Could you check a few things on this model? Use its own coordinates, in mm. A direction names the side the tool comes from. Round coordinates to 2 decimals unless told otherwise and drop trailing zeros. One line per question, with ' | ' between items. Start each with the question number.
1. If I drill on line 1 along Y through (x, z) = (80, 16); line 2 along Y through (x, z) = (-80, 14); line 3 along Z through (x, y) = (34, -32), over which ranges is the centre line in solid material (lowest first)? Write a range as [from, to].
2. For pin 1 Ø3 at (x, y) = (0, -80) entering from -Z; pin 2 Ø3 at (x, z) = (-57.5, 9) entering from -Y; pin 3 Ø8 at (y, z) = (22.5, 12.5) entering from +X; pin 4 Ø18 at (x, y) = (2, -5.5) entering from -Z, each with a flat end and sliding along its axis, tell me the tip position at first contact or that it passes through.
3. Thinking about a two-plate mould opening in Y: for faces 1 (the flat face through (-80.1, 2.2, 0)), 2 (the cylindrical face through (-75.381, 1.915, 14.61)), 3 (the conical face through (-94.395, -29.726, 5.804)), which applies, released by +Y, released by -Y, zero draft, split by the parting line, or undercut?
4. For faces 4 (the cylindrical face through (75, 0, 15)), 5 (the conical face through (-14.037, 5.82, 5.582)), which set-ups out of +Z, -Z, +X, -X, +Y, -Y let a thin tool reach every point of the face, with its end or its side?
from build123d import *

# Parameters (mm, degrees)
F2_R   = 5
F2_R_2 = 2


with BuildPart() as f1:
    # F0 (on Front) → F1 (revolve)
    with BuildSketch(Plane.XZ):
        with BuildLine():
            Line((-46.5626491532, 34.7380191088), (-64.5524207617, 34.7380191088))
            ThreePointArc((-64.5524207617, 34.7380191088), (-74.4188193129, 33.0691712144), (-83.1875166342, 28.2482977508))
            Line((-83.1875166342, 28.2482977508), (-87.9970200386, 24.436111668))
            ThreePointArc((-87.9970200386, 24.436111668), (-95.1163936469, 16.3111280107), (-98.8962470082, 6.1911700773))
            Line((-98.8962470082, 6.1911700773), (-100, 0))
            Line((-100, 0), (-96.9526980361, 0))
            Line((-96.9526980361, 0), (-95.942814724, 5.6646363721))
            ThreePointArc((-95.942814724, 5.6646363721), (-92.5409466988, 14.7725985122), (-86.1335104514, 22.0850838038))
            Line((-86.1335104514, 22.0850838038), (-81.324007047, 25.8972698866))
            ThreePointArc((-81.324007047, 25.8972698866), (-73.4321794578, 30.2360560038), (-64.5524207617, 31.7380191088))
            Line((-64.5524207617, 31.7380191088), (-46.5626491532, 31.7380191088))
            ThreePointArc((-46.5626491532, 31.7380191088), (-30.80440398, 26.6623824761), (-20.9708348415, 13.3437753355))
            Line((-20.9708348415, 13.3437753355), (-18.1650745435, 5))
            Line((-18.1650745435, 5), (-15, 5))
            Line((-15, 5), (-18.1272999179, 14.2999704719))
            ThreePointArc((-18.1272999179, 14.2999704719), (-29.0534878496, 29.0984228502), (-46.5626491532, 34.7380191088))
        make_face()
    revolve(axis=Axis((0, 0, 26.7854109406), (0, 0, 1)))

    # F2 (on face) → F3 (join, up to the next surface of F1)
    with BuildSketch(Plane(origin=(0, 0, 0), x_dir=(1, 0, 0), z_dir=(0, 0, -1))):
        with Locations((80, 0)):
            Circle(F2_R)
        with Locations((80, 0)):
            Circle(F2_R_2, mode=Mode.SUBTRACT)
        with Locations((0, 80)):
            Circle(F2_R)
        with Locations((0, 80)):
            Circle(F2_R_2, mode=Mode.SUBTRACT)
        with Locations((-80, 0)):
            Circle(F2_R)
        with Locations((-80, 0)):
            Circle(F2_R_2, mode=Mode.SUBTRACT)
        with Locations((0, -80)):
            Circle(F2_R)
        with Locations((0, -80)):
            Circle(F2_R_2, mode=Mode.SUBTRACT)
    extrude(until=Until.NEXT, dir=(0, 0, 1))


solid = f1.part
Geometry results:
1) line 1: y = [-51.79, -44.95], [-5, -2], [2, 5], [44.95, 51.79] | line 2: y = [-53.72, -47.39], [-5, -2], [2, 5], [47.39, 53.72] | line 3: z = [31.74, 34.74]
2) pin 1: stops at z = 25.76 | pin 2: stops at y = -80.84 | pin 3: stops at x = 96.09 | pin 4: passes through
3) face 1: zero draft | face 2: undercut | face 3: split by the parting line
4) face 4: -Z | face 5: +Z
